Model file for the job. Use its own axes, mm. Face numbers are marked on the shaded views. A direction names the side the tool comes from. Give positions to 0.01 mm unless a question says otherwise; leave off trailing zeros. Loops run counter-clockwise (first coordinate to the right, second up) from the corner with the lowest first, then second, coordinate; pieces in that order, holes last. Notation, with made-up numbers: M 53,87.25 L 62,87.25 A16 ccw 62,104.25 Z; hole C 46,35 d1. An arc over 180 degrees is marked long. Answer in a Markdown table with one row per item.
Autodesk Inventor part; units mm, degrees
ref_plane "YZ Plane" through (0, 0, 0) normal (1, 0, 0) x (0, 1, 0)
ref_plane "XZ Plane" through (0, 0, 0) normal (0, 1, 0) x (-1, 0, 0)
ref_plane "XY Plane" through (0, 0, 0) normal (0, 0, 1) x (1, 0, 0)
sketch "Sketch1" plane through (0, 0, 0) normal (0, 0, 1) x (1, 0, 0)
  line L0 (6.35, 28.575) -> (25.4, 28.575)
  line L1 (6.35, 31.75) -> (25.4, 31.75)
  line L2 (25.4, 0) -> (6.35, 0)
  arc A0 (0, 6.35) -> (6.35, 0) centre (6.35, 6.35) ccw
  line L3 (0, 6.35) -> (0, 25.4)
  arc A1 (6.35, 31.75) -> (0, 25.4) centre (6.35, 25.4) ccw
  line L4 (6.35, 31.75) -> (25.4, 31.75)
  line L5 (25.4, 28.575) -> (6.35, 28.575)
  arc A2 (6.35, 28.575) -> (3.175, 25.4) centre (6.35, 25.4) ccw
  line L6 (3.175, 25.4) -> (3.175, 6.35)
  arc A3 (3.175, 6.35) -> (6.35, 3.175) centre (6.35, 6.35) ccw
  line L7 (6.35, 3.175) -> (25.4, 3.175)
  line L8 (28.575, 3.175) -> (28.575, 0)
  line L9 (25.4, 31.75) -> (28.575, 31.75)
  line L10 (28.575, 28.575) -> (25.4, 28.575)
  line L11 (28.575, 31.75) -> (28.575, 28.575)
  line L12 (28.575, 0) -> (25.4, 0)
  line L13 (28.575, 3.175) -> (28.575, 0)
  line L14 (25.4, 3.175) -> (28.575, 3.175)
  point P0 (0, 0)
extrude "Extrusion1" add sketch "Sketch1" against normal blind 762
chamfer "Chamfer1" distance 3.175 angle 45 4 edges at (28.575, 30.1625, 0) (28.575, 1.5875, 0) (28.575, 30.1625, -762) (28.575, 1.5875, -762)
sketch "Sketch2" plane through (6.35, 31.75, 0) normal (0, 1, 0) x (1, 0, 0)
  line L0 (19.05, 0) -> (0, 0)
  line L1 (22.225, 3.175) -> (22.225, 758.825)
  point P0 (-6.35, 0)
  point P1 (9.525, 12.7)
  dimension "d5" = 12.7
  dimension "d6" = 12.7
hole "Hole1" at (15.875, 31.75, -12.7) direction (0, -1, 0) diameter 6.7056 end through all
pattern_linear "Rectangular Pattern1" count 30 spacing 25.4 along (0, 0, -1) of "Hole1"
sketch "Sketch3" plane through (0, 6.35, 0) normal (-1, 0, 0) x (0, 0, 1)
  line L0 (-0.2722, 19.0092) -> (-759.0056, 19.0092)
  line L1 (-759.0056, 19.0092) -> (-759.0056, 0.0408)
  line L2 (-0.2722, 0.0408) -> (-759.0056, 0.0408)
  line L3 (-0.2722, 0.0408) -> (-0.2722, 19.0092)
  circle A0 centre (-698.5852, 9.525) radius 4.78
  circle A1 centre (-111.2243, 9.525) radius 4.78
  circle A2 centre (-188.7416, 9.525) radius 3.6672
  circle A3 centre (-277.2605, 9.525) radius 3.6672
  circle A4 centre (-481.9921, 9.525) radius 3.6672
  circle A5 centre (-570.511, 9.525) radius 3.6672
  circle A6 centre (-469.3591, 9.525) radius 3.6672
  circle A7 centre (-583.1692, 9.525) radius 3.6672
  circle A8 centre (-289.9187, 9.525) radius 3.6672
  circle A9 centre (-176.1087, 9.525) radius 3.6672
  circle A10 centre (-551.6311, 9.525) radius 4.78
  circle A11 centre (-526.34, 9.525) radius 4.78
  circle A12 centre (-501.0489, 9.525) radius 4.78
  circle A13 centre (-258.2289, 9.525) radius 4.78
  circle A14 centre (-232.9378, 9.525) radius 4.78
  circle A15 centre (-207.6467, 9.525) radius 4.78
  circle A16 centre (-607.2589, 9.525) radius 1.5807
  circle A17 centre (-152.0189, 9.525) radius 1.5807
  circle A18 centre (-379.6389, 5.9842) radius 4.78
  circle A19 centre (-85.9332, 9.525) radius 4.78
  circle A20 centre (-673.294, 9.525) radius 4.78
  circle A21 centre (-648.0029, 9.525) radius 4.78
  circle A22 centre (-63.5, 9.525) radius 4.8006
  point P0 (0, -6.35)
  point P1 (-759.0056, -6.2819)
  dimension "d21" = 9.6012
extrude "Extrusion2" [suppressed]
sketch "Sketch4" plane through (6.35, 31.75, 0) normal (0, 1, 0) x (1, 0, 0)
  line L0 (-18.2452, 129.5546) -> (88.0083, 129.5546)
  line L1 (88.0083, 129.5546) -> (88.0083, 1027.7541)
  line L2 (88.0083, 1027.7541) -> (-18.2452, 1027.7541)
  line L3 (-18.2452, 1027.7541) -> (-18.2452, 129.5546)
  point P0 (-6.35, 0)
extrude "Extrusion3" cut sketch "Sketch4" against normal blind 50.8
sketch "Sketch5" plane through (0, 6.35, 0) normal (-1, 0, 0) x (0, 0, 1)
  circle A0 centre (-63.5, 9.525) radius 4.8006
  dimension "d23" = 9.6012
extrude "Extrusion4" cut sketch "Sketch5" against normal through all
properties part number "am-2222" material "Aluminum 6061"
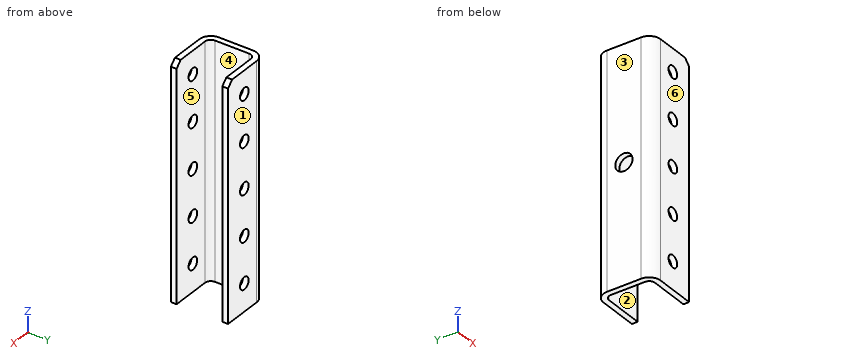
(1) Which spindle directions (+Z, -Z, +X, -X, +Y, -Y) get a long thin tool onto all of the face, cutting with end or side? Do the marked faces 1 and 2. Say none if no direction does.
Established:
| item | result |
|---|---|
| face 1 | +Z, -Z, +X, -X, +Y |
| face 2 | +Z, -Z, +X |
(2) Saw through at C-C, the plane z = -114.3. Give the cut face in (x, y) (3 decimals).
Established:
| item | result |
|---|---|
| outline | M 0,6.35 A6.35 ccw 6.35,0 L 12.522,0 L 12.522,3.175 L 6.35,3.175 A3.175 cw 3.175,6.35 L 3.175,25.4 A3.175 cw 6.35,28.575 L 12.522,28.575 L 12.522,31.75 L 6.35,31.75 A6.35 ccw 0,25.4 Z; M 19.228,0 L 28.575,0 L 28.575,3.175 L 19.228,3.175 Z; M 19.228,28.575 L 28.575,28.575 L 28.575,31.75 L 19.228,31.75 Z |
(3) Saw through at B-B, the plane x = 21. Give the cut face in (y, z) (3 decimals), and give its area (3 significant figures).
Established:
| item | result |
|---|---|
| outline | M 0,-129.555 L 3.175,-129.555 L 3.175,0 L 0,0 Z; M 28.575,-129.555 L 31.75,-129.555 L 31.75,0 L 28.575,0 Z |
| area | 823 mm2 |
(4) Saw through at D-D, the plane z = -101. Give the cut face in (x, y) (3 decimals), and give its area (3 significant figures).
Established:
| item | result |
|---|---|
| outline | M 0,6.35 A6.35 ccw 6.35,0 L 28.575,0 L 28.575,3.175 L 6.35,3.175 A3.175 cw 3.175,6.35 L 3.175,25.4 A3.175 cw 6.35,28.575 L 28.575,28.575 L 28.575,31.75 L 6.35,31.75 A6.35 ccw 0,25.4 Z |
| area | 249 mm2 |
(5) Mould opens along Y. For the marked faces 3, 4, 5 and 6 say: pulls with the +Y half, pulls with the -Y half, needs draft (parallel to the pull), parting line crosses it, or undercut.
Established:
| item | result |
|---|---|
| face 3 | needs draft |
| face 4 | undercut |
| face 5 | undercut |
| face 6 | pulls with the -Y half |
(6) Saw through at A-A, the plane z = -63.5. Give the cut face in (x, y) (3 decimals).
Established:
| item | result |
|---|---|
| outline | M 0,6.35 A6.35 ccw 6.35,0 L 12.522,0 L 12.522,3.175 L 6.35,3.175 A3.175 cw 3.175,6.35 L 3.175,11.074 L 0,11.074 Z; M 0,20.676 L 3.175,20.676 L 3.175,25.4 A3.175 cw 6.35,28.575 L 12.522,28.575 L 12.522,31.75 L 6.35,31.75 A6.35 ccw 0,25.4 Z; M 19.228,0 L 28.575,0 L 28.575,3.175 L 19.228,3.175 Z; M 19.228,28.575 L 28.575,28.575 L 28.575,31.75 L 19.228,31.75 Z |
(7) Flat gauge pins, fed straight in: P1, Ø5.5, axis at x = 15.875, z = -38.1, coming from the +Y side; P2, Ø10.5, axis at x = 15.875, z = -114.3, coming from the +Y side; P3, Ø9.5, axis at y = 13, z = -75, coming from the +X side (3 decimals). Where does each tip first touch, or does it go through?
Established:
| item | result |
|---|---|
| P1 | passes through |
| P2 | stops at y = 31.75 |
| P3 | stops at x = 3.175 |
(8) Wall check: L1, parallel to Y at x = 26, z = -54.5 (3 decimals); L2, parallel to Z at x = 17, y = 2.5; L3, parallel to X at y = 31, z = -12.7 (3 decimals). Give the ranges that are in metal, low to high.
Established:
| item | result |
|---|---|
| L1 | y = 0 to 3.175, 28.575 to 31.75 |
| L2 | z = -129.55 to -117.46, -111.14 to -92.06, -85.74 to -66.66, -60.34 to -41.26, -34.94 to -15.86, -9.54 to 0 |
| L3 | x = 3.356 to 12.522, 19.228 to 28.575 |
